from build123d import *

# Parameters (mm, degrees)
F0_W         = 90
F0_H         = 33
F0_R         = 1.5
F1_DEPTH     = 2
F2_W         = 5
F2_H         = 33
F3_DEPTH     = 27.5
F4_W         = 2
F4_H         = 33
F5_DEPTH     = 25
F6_W         = 2
F6_H         = 33
F7_DEPTH     = 25
F9_D         = 3.4
F10_R        = 5
F11_SIZE     = 12
F12_T1_DEPTH = 27.1366974606


# Not quite as in the source:
# - a fillet or chamfer that OpenCascade refuses, or shapes differently, is made with other operations: its cross-section is extruded or revolved along the edge and cut away or added


with BuildPart() as f1:
    # F0 (on Top) → F1 (new body)
    with BuildSketch(Plane.XY):
        Rectangle(F0_W, F0_H)
        with Locations((-40.91, 0)):
            Circle(F0_R, mode=Mode.SUBTRACT)
        with Locations((40.91, 0)):
            Circle(F0_R, mode=Mode.SUBTRACT)
    extrude(amount=F1_DEPTH)

    # F2 (on face) → F3 (join)
    with BuildSketch(Plane.XY.offset(2)):
        with Locations((-29.5, 0)):
            Rectangle(F2_W, F2_H)
        with Locations((29.5, 0)):
            Rectangle(F2_W, F2_H)
    extrude(amount=F3_DEPTH)

    # F4 (on face) → F5 (join)
    with BuildSketch(Plane.XY.offset(29.5)):
        with Locations((-31, 0)):
            Rectangle(F4_W, F4_H)
    extrude(amount=F5_DEPTH)

    # F6 (on face) → F7 (join)
    with BuildSketch(Plane.XY.offset(29.5)):
        with Locations((31, 0)):
            Rectangle(F6_W, F6_H)
    extrude(amount=F7_DEPTH)

    # F9 (through all)
    with Locations(Plane(origin=(-32, 0, 0), x_dir=(0, -1, 0), z_dir=(-1, 0, 0))):
        with Locations((-10, 47), (-10, 39.5), (0, 39.5), (0, 47), (10, 47), (10, 39.5), (-10, 32), (0, 32), (10, 32)):
            Hole(F9_D / 2)

    # F10
    f10_edges = [f1.edges().sort_by_distance(p)[0] for p in [
        (-31, 16.5, 54.5),
        (31, 16.5, 54.5),
        (-31, -16.5, 54.5),
        (31, -16.5, 54.5),
    ]]
    fillet(f10_edges, radius=F10_R)

    # F11
    f11_edges = [f1.edges().sort_by_distance(p)[0] for p in [
        (45, 16.5, 1),
        (45, -16.5, 1),
        (-45, -16.5, 1),
        (-45, 16.5, 1),
    ]]
    chamfer(f11_edges, length=F11_SIZE)

    # F12: fillet of radius 12.1370711845 on 4 edges, made by hand

    # F12_s2 → F12_t1 (cut)
    with BuildSketch(Plane.XY.offset(-12.5683487303)):
        with BuildLine():
            ThreePointArc((41.4451341538, -8.0548658462), (44.0761204675, -4.1173165676), (45, 0.5273394921))
            Line((45, 0.5273394921), (45, -4.5))
            Line((45, -4.5), (41.4451341538, -8.0548658462))
        make_face()
        with BuildLine():
            ThreePointArc((45, -0.5273394921), (44.0761204675, 4.1173165676), (41.4451341538, 8.0548658462))
            Line((41.4451341538, 8.0548658462), (45, 4.5))
            Line((45, 4.5), (45, -0.5273394921))
        make_face()
        with BuildLine():
            ThreePointArc((-41.4451341538, -8.0548658462), (-44.0761204675, -4.1173165676), (-45, 0.5273394921))
            Line((-45, 0.5273394921), (-45, -4.5))
            Line((-45, -4.5), (-41.4451341538, -8.0548658462))
        make_face()
        with BuildLine():
            ThreePointArc((-45, -0.5273394921), (-44.0761204675, 4.1173165676), (-41.4451341538, 8.0548658462))
            Line((-41.4451341538, 8.0548658462), (-45, 4.5))
            Line((-45, 4.5), (-45, -0.5273394921))
        make_face()
    extrude(amount=F12_T1_DEPTH, mode=Mode.SUBTRACT)


solid = f1.part
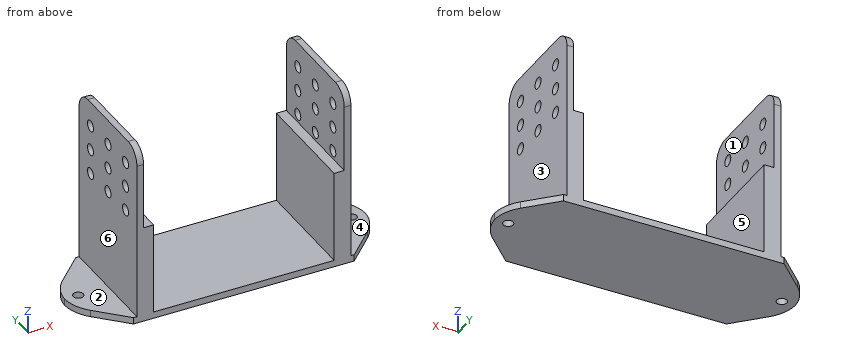
The model under review builds one solid part; all positions refer to its coordinate system, in mm. Face numbers are marked on the shaded views. A direction names the side the tool comes from. Coordinates: 2 decimals unless noted, no trailing zeros. Order: outer loops, then holes, each group sorted by start corner. A loop starts at its lowest first (then second) coordinate and runs counter-clockwise, first axis right, second up. Notation, with made-up numbers: (34, -14.75) -> (43, -14.75) arc R30 cw to (43, 16.25) -> close; hole circle Ø3 at (85.5, 34). An arc over 180 degrees is marked (long way). Answer in a Markdown table with one row per item.
(1) Wall thickness on line 1 along Z through (x, y) = (31, 0); line 2 along X through (y, z) = (0, 41.5); line 3 along X through (y, z) = (3, 5): over which ranges is each line inside the solid? List them lowest first.
Answers:
| item | result |
|---|---|
| line 1 | 0 to 30.3, 33.7 to 37.8, 41.2 to 45.3, 48.7 to 54.5 |
| line 2 | -32 to -30, 30 to 32 |
| line 3 | -32 to -27, 27 to 32 |
(2) Consider section D-D (x = 37.5). Write out the cut boundary in (y, z).
Answers:
| item | result |
|---|---|
| outline | (-12, 0) -> (12, 0) -> (12, 2) -> (-12, 2) -> close |
(3) Consider section B-B (y = -10). State how many separate pieces and enclosed holes the cut face has, plus the area to 3 significant figures.
Answers:
| item | result |
|---|---|
| separate pieces | 7 |
| enclosed holes | 0 |
| area | 492 mm² |
(4) Consider section C-C (z = 6.5). Write out the cut boundary in (x, y).
Answers:
| item | result |
|---|---|
| outline | (-32, -16.5) -> (-27, -16.5) -> (-27, 16.5) -> (-32, 16.5) -> close; (27, -16.5) -> (32, -16.5) -> (32, 16.5) -> (27, 16.5) -> close |
(5) Machinability: for the marked faces 1, 2 and 3, which of the approach directions +Z, -Z, +X, -X, +Y, -Y give a long, thin tool a straight path to every point of the face, cutting with its end or side? Answer none if there is none.
Answers:
| item | result |
|---|---|
| face 1 | +Z, +Y, -Y |
| face 2 | +Z, -X, +Y, -Y |
| face 3 | +Z, +X, +Y, -Y |
(6) Consider section A-A (z = 43). Write out the cut boundary in (x, y).
Answers:
| item | result |
|---|---|
| outline | (-32, -16.5) -> (-30, -16.5) -> (-30, 16.5) -> (-32, 16.5) -> close; (30, -16.5) -> (32, -16.5) -> (32, 16.5) -> (30, 16.5) -> close |
(7) Insertion check: pin 1 (6 mm diameter, centred on x = -21.5, y = 8, fed in from +Z); pin 2 (12 mm diameter, centred on y = -11, z = 38.5, fed in from +X); pin 3 (3.5 mm diameter, centred on x = 29, y = 2, fed in from +Z); pin 4 (5 mm diameter, centred on y = -9, z = 28.5, fed in from -X). Each pin has a flat end and moves straight along its axis. Give the tip position at first contact, or say it passes through.
Answers:
| item | result |
|---|---|
| pin 1 | z = 2 |
| pin 2 | x = 32 |
| pin 3 | z = 54.5 |
| pin 4 | x = -32 |
(8) The part is to be moulded in two halves that separate along X. For the marked faces 4, 5 and 6, say which applies: +X half, -X half, draft (parallel to the pull), parting line (faces both ways), or undercut.
Answers:
| item | result |
|---|---|
| face 4 | draft |
| face 5 | undercut |
| face 6 | -X half |
